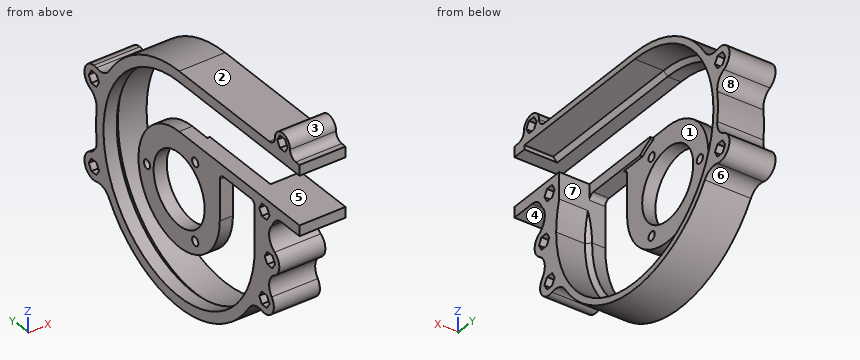
```python
from build123d import *

# Parameters (mm, degrees)
SKETCH_2_W           = 17.5
SKETCH_2_H           = 4
EXTRUDE_1_DEPTH      = 6
SKETCH_6_R           = 13.5
SKETCH_6_R_2         = 1.65
EXTRUDE_2_DEPTH      = 5
FILLET_1_R           = 2
EXTRUDE_START        = -17.5
SKETCH_7_R           = 5
EXTRUDE_3_DEPTH      = 17.5
FILLET_2_R           = 6
CUT_EXTRUDE_1_DEPTH  = 72.072146443
SKETCH_9_W           = 17.5
SKETCH_9_H           = 4
EXTRUDE_4_DEPTH      = 11.4
FILLET_3_R           = 5
EXTRUDE_5_DEPTH      = 0.28
EXTRUDE_5_DEPTH_BACK = 5
SKETCH_10_W          = 17.5
SKETCH_10_H          = 4
SKETCH_11_R          = 4
EXTRUDE_6_DEPTH      = 17.5
FILLET_4_R           = 3


with BuildPart() as part:
    # Sweep 1: sweep along a path in 草图1
    with BuildLine(Plane(origin=(0, 0, 0), x_dir=(0, 0, -1), z_dir=(1, 0, 0))) as sweep_1_path:
        Line((-44, -52), (-44, 0))
        ThreePointArc((-44, 0), (31.112698372, 31.112698372), (0, -44))
        Line((0, -44), (-17.5, -44))
        Line((-17.5, -44), (-17.5, -52))
    # 草图2 → Sweep 1 (sweep)
    with BuildSketch(Plane(origin=(0, -52, 0), x_dir=(1, 0, 0), z_dir=(0, 1, 0))):
        with Locations((8.75, -42)):
            Rectangle(SKETCH_2_W, SKETCH_2_H)
    sweep(path=sweep_1_path.line, transition=Transition.RIGHT)

    # Sweep 1 2: sweep along a path in 草图4
    with BuildLine(Plane.ZY) as sweep_1_2_path:
        Line((44, -52), (44, 0))
        ThreePointArc((44, 0), (-31.112698372, 31.112698372), (0, -44))
        ThreePointArc((0, -44), (12.692125838, -42.129680057), (24.3052364, -36.677724623))
    # 草图3 → Sweep 1 2 (sweep, cut)
    with BuildSketch(Plane(origin=(0, -52, 0), x_dir=(1, 0, 0), z_dir=(0, 1, 0))):
        Polygon((17.5, -40), (5, -40), (6.6, -41.6), (17.5, -41.6), align=None)
    sweep(path=sweep_1_2_path.line, mode=Mode.SUBTRACT)

    # 草图5 → 凸台-拉伸1 (add)
    with BuildSketch(Plane.ZY):
        with BuildLine():
            Line((21.5, -40), (21.5, -8.077747211))
            ThreePointArc((21.5, -8.077747211), (21.091287093, -7.586151171), (20.533333333, -7.898241717))
            ThreePointArc((20.533333333, -7.898241717), (19.209784895, -10.723066925), (17.5, -13.332291626))
            Line((17.5, -13.332291626), (17.5, -40))
            Line((17.5, -40), (21.5, -40))
        make_face()
    extrude(amount=-EXTRUDE_1_DEPTH)

    # 草图6 → 凸台-拉伸2 (add)
    with BuildSketch(Plane.ZY):
        with BuildLine():
            Line((21.5, -21.5), (21.5, -8.077747211))
            Line((21.5, -8.077747211), (21.5, 0))
            ThreePointArc((21.5, 0), (-15.202795796, 15.202795796), (0, -21.5))
            Line((0, -21.5), (21.5, -21.5))
        make_face()
        Circle(SKETCH_6_R, mode=Mode.SUBTRACT)
        with Locations((0, 17)):
            Circle(SKETCH_6_R_2, mode=Mode.SUBTRACT)
        with Locations((14.722431864, -8.5)):
            Circle(SKETCH_6_R_2, mode=Mode.SUBTRACT)
        with Locations((-14.722431864, -8.5)):
            Circle(SKETCH_6_R_2, mode=Mode.SUBTRACT)
    extrude(amount=-EXTRUDE_2_DEPTH)

    # 圆角1
    fillet_1_edges = [part.edges().sort_by_distance(p)[0] for p in [
        (3, -40, 17.5),
        (2.5, -21.5, 17.5),
    ]]
    fillet(fillet_1_edges, radius=FILLET_1_R)

    # 草图7 → 凸台-拉伸3 (add)
    # profile 1 of 7: a face of its own
    with BuildSketch(Plane.ZY.offset(EXTRUDE_START)):
        with BuildLine():
            ThreePointArc((-11.41696688, -45.105245798), (-11.647855738, -43.60338731), (-12.319198447, -42.240233778))
            ThreePointArc((-12.319198447, -42.240233778), (-15.048886306, -41.346475315), (-17.714445389, -40.276524485))
            ThreePointArc((-17.714445389, -40.276524485), (-20.865936265, -47.387058983), (-13.252416867, -48.976372665))
            ThreePointArc((-13.252416867, -48.976372665), (-11.899071902, -47.247353398), (-11.41696688, -45.105245798))
        make_face()
        Polygon((-14.06696688, -46.46201893), (-16.41696688, -47.818792063), (-18.76696688, -46.46201893), (-18.76696688, -43.748472665), (-16.41696688, -42.391699533), (-14.06696688, -43.748472665), align=None, mode=Mode.SUBTRACT)
    # profile 2 of 7: a face of its own
    with BuildSketch(Plane.ZY.offset(EXTRUDE_START)):
        with BuildLine():
            ThreePointArc((-4.29770766, -50.555329502), (-4.888687372, -46.950840441), (-2.870750936, -43.90625))
            ThreePointArc((-2.870750936, -43.90625), (-7.640519817, -43.331541133), (-12.319198447, -42.240233778))
            ThreePointArc((-12.319198447, -42.240233778), (-11.647855738, -43.60338731), (-11.41696688, -45.105245798))
            ThreePointArc((-11.41696688, -45.105245798), (-11.899071902, -47.247353398), (-13.252416867, -48.976372665))
            ThreePointArc((-13.252416867, -48.976372665), (-8.413067787, -47.712878387), (-4.29770766, -50.555329502))
        make_face()
    # profile 3 of 7: a face of its own
    with BuildSketch(Plane.ZY.offset(EXTRUDE_START)):
        with BuildLine():
            ThreePointArc((5, -48), (4.472135955, -45.763932023), (3, -44))
            ThreePointArc((3, -44), (1.58113883, -43.25658351), (0, -43))
            Line((0, -43), (0, -44))
            ThreePointArc((0, -44), (-1.436140662, -43.976556254), (-2.870750936, -43.90625))
            ThreePointArc((-2.870750936, -43.90625), (-4.888687372, -46.950840441), (-4.29770766, -50.555329502))
            ThreePointArc((-4.29770766, -50.555329502), (0, -53), (4.29770766, -50.555329502))
            ThreePointArc((4.29770766, -50.555329502), (4.821231083, -49.325039942), (5, -48))
        make_face()
        Polygon((-2.35, -46.643226867), (0, -45.286453735), (2.35, -46.643226867), (2.35, -49.356773133), (0, -50.713546265), (-2.35, -49.356773133), align=None, mode=Mode.SUBTRACT)
    # profile 4 of 7: a face of its own
    with BuildSketch(Plane.ZY.offset(EXTRUDE_START)):
        with BuildLine():
            Line((11.540653546, -44), (3, -44))
            ThreePointArc((3, -44), (4.472135955, -45.763932023), (5, -48))
            ThreePointArc((5, -48), (4.821231083, -49.325039942), (4.29770766, -50.555329502))
            ThreePointArc((4.29770766, -50.555329502), (8.413067787, -47.712878387), (13.252416867, -48.976372665))
            ThreePointArc((13.252416867, -48.976372665), (11.688865563, -46.731609207), (11.540653546, -44))
        make_face()
    # profile 5 of 7: a face of its own
    with BuildSketch(Plane.ZY.offset(EXTRUDE_START)):
        with Locations((16.41696688, -45.105245798)):
            Circle(SKETCH_7_R)
        Polygon((18.76696688, -46.46201893), (16.41696688, -47.818792063), (14.06696688, -46.46201893), (14.06696688, -43.748472665), (16.41696688, -42.391699533), (18.76696688, -43.748472665), align=None, mode=Mode.SUBTRACT)
    # profile 6 of 7: a face of its own
    with BuildSketch(Plane.ZY.offset(EXTRUDE_START)):
        with BuildLine():
            ThreePointArc((-11.41696688, 45.105245798), (-19.459384295, 49.07307849), (-17.714445389, 40.276524485))
            ThreePointArc((-17.714445389, 40.276524485), (-15.048886306, 41.346475315), (-12.319198447, 42.240233778))
            ThreePointArc((-12.319198447, 42.240233778), (-11.647855738, 43.60338731), (-11.41696688, 45.105245798))
        make_face()
        Polygon((-18.76696688, 43.748472665), (-18.76696688, 46.46201893), (-16.41696688, 47.818792063), (-14.06696688, 46.46201893), (-14.06696688, 43.748472665), (-16.41696688, 42.391699533), align=None, mode=Mode.SUBTRACT)
    # profile 7 of 7: a face of its own
    with BuildSketch(Plane.ZY.offset(EXTRUDE_START)):
        with BuildLine():
            ThreePointArc((21.41696688, 45.105245798), (14.915108391, 49.874356939), (12.319198447, 42.240233778))
            ThreePointArc((12.319198447, 42.240233778), (15.048886306, 41.346475315), (17.714445389, 40.276524485))
            ThreePointArc((17.714445389, 40.276524485), (20.384799572, 42.062828383), (21.41696688, 45.105245798))
        make_face()
        Polygon((14.06696688, 46.46201893), (16.41696688, 47.818792063), (18.76696688, 46.46201893), (18.76696688, 43.748472665), (16.41696688, 42.391699533), (14.06696688, 43.748472665), align=None, mode=Mode.SUBTRACT)
    extrude(amount=EXTRUDE_3_DEPTH)

    # 圆角2
    # the kernel refuses this fillet: 6 mm, written as the material it adds along each edge
    with BuildSketch(Plane(origin=(17.5, 40.276524485, -17.714445389), x_dir=(0, -0.4726837072692949, -0.8812321560645388), z_dir=(-1, 0, 0)), Plane(origin=(17.5, 42.240233778, 12.319198447), x_dir=(0, 0.20434838386912327, -0.978898226584397), z_dir=(-1, 0, 0))) as fillet_2_piece_1:
        with BuildLine():
            CenterArc((7.322424831, -5.98176794), FILLET_2_R, 94.467760731, 73.250864603)
            Line((1.459736191, -4.705491359), (1.342482418, -4.679965828))
            ThreePointArc((1.342482418, -4.679965828), (1.235040355, -2.196031285), (-0.082220104, -0.087406261))
            Line((-0.082220104, -0.087406261), (0.009347776, 0.119635359))
            ThreePointArc((0.009347776, 0.119635359), (3.427518006, -0.013701771), (6.845688236, 0.119635359))
            Line((6.845688236, 0.119635359), (6.855036012, 0))
        make_face()
    extrude(amount=17.5)
    with BuildSketch(Plane(origin=(17.5, 42.240233778, -12.319198447), x_dir=(0, 0.20434838386906956, 0.9788982265844082), z_dir=(-1, 0, 0)), Plane(origin=(17.5, 40.276524485, 17.714445389), x_dir=(0, -0.47268370726929204, 0.8812321560645403), z_dir=(-1, 0, 0)), Plane(origin=(17.5, -40.276524485, -17.714445389), x_dir=(0, 0.47268370726929143, -0.8812321560645405), z_dir=(-1, 0, 0))) as fillet_2_piece_2:
        with BuildLine():
            CenterArc((7.322424831, 5.98176794), FILLET_2_R, 192.281374666, 73.250864603)
            Line((1.459736191, 4.705491359), (1.342482418, 4.679965828))
            ThreePointArc((1.342482418, 4.679965828), (1.235040355, 2.196031285), (-0.082220104, 0.087406261))
            Line((-0.082220104, 0.087406261), (0.009347776, -0.119635359))
            ThreePointArc((0.009347776, -0.119635359), (3.427518006, 0.013701771), (6.845688236, -0.119635359))
            Line((6.845688236, -0.119635359), (6.855036012, 0))
        make_face()
    extrude(amount=17.5)
    with BuildSketch(Plane(origin=(0, -49.986540632, 17.5), x_dir=(0, -1, 0), z_dir=(1, 0, 0))) as fillet_2_piece_3:
        with BuildLine():
            CenterArc((5.420881339, 4.938570189), FILLET_2_R, 200.518106547, 34.877722735)
            Line((-0.198487483, 2.83554997), (-0.310874859, 2.793489565))
            ThreePointArc((-0.310874859, 2.793489565), (-0.013206953, 1.423797529), (-0.117151076, 0.025992795))
            Line((-0.117151076, 0.025992795), (0, -0.12))
            ThreePointArc((0, -0.12), (1.006729684, -0.12), (1.945310928, -0.098771404))
            Line((1.945310928, -0.098771404), (2.013459368, 0))
        make_face()
    extrude(amount=17.5)

    # 草图8 → 切除-拉伸1 (cut, through all)
    with BuildSketch(Plane(origin=(17.5, 0, 0), x_dir=(0, 0, -1), z_dir=(1, 0, 0))):
        Polygon((-14.06696688, -46.46201893), (-14.06696688, -43.748472665), (-16.41696688, -42.391699533), (-18.76696688, -43.748472665), (-18.76696688, -46.46201893), (-16.41696688, -47.818792063), align=None)
    extrude(amount=-CUT_EXTRUDE_1_DEPTH, mode=Mode.SUBTRACT)

    # 草图9 → 凸台-拉伸4 (add)
    with BuildSketch(Plane.XZ.offset(52)):
        with Locations((8.75, 19.5)):
            Rectangle(SKETCH_9_W, SKETCH_9_H)
        Polygon((6.6, 41.6), (17.5, 41.6), (17.5, 44), (0, 44), (0, 40), (5, 40), align=None)
    extrude(amount=EXTRUDE_4_DEPTH)

    # 圆角3
    fillet_3_edges = [part.edges().sort_by_distance(p)[0] for p in [
        (8.75, -52, 17.5),
    ]]
    fillet(fillet_3_edges, radius=FILLET_3_R)

    # 草图10 → 凸台-拉伸5 (add, two sides: drawn at the far end of the back side and taken through both)
    with BuildSketch(Plane.XZ.offset(63.4).offset(-EXTRUDE_5_DEPTH_BACK)):
        with Locations((8.75, 42)):
            Rectangle(SKETCH_10_W, SKETCH_10_H)
        with Locations((8.75, 19.5)):
            Rectangle(SKETCH_10_W, SKETCH_10_H)
    extrude(amount=EXTRUDE_5_DEPTH + EXTRUDE_5_DEPTH_BACK)

    # 草图11 → 凸台-拉伸6 (add)
    with BuildSketch(Plane(origin=(17.5, 0, 0), x_dir=(0, 0, -1), z_dir=(1, 0, 0))):
        with Locations((-47, -54.68)):
            Circle(SKETCH_11_R)
        Polygon((-44.65, -53.323226867), (-47, -51.966453735), (-49.35, -53.323226867), (-49.35, -56.036773133), (-47, -57.393546265), (-44.65, -56.036773133), align=None, mode=Mode.SUBTRACT)
    extrude(amount=-EXTRUDE_6_DEPTH)

    # 圆角4
    fillet_4_edges = [part.edges().sort_by_distance(p)[0] for p in [
        (8.75, -52.034248689, 44),
        (8.75, -57.325751311, 44),
    ]]
    fillet(fillet_4_edges, radius=FILLET_4_R)


solid = part.part
```
For this review, take the finished solid that the model builds, in its own axes (mm). Face numbers are marked on the shaded views. A direction names the side the tool comes from. Give positions to 0.01 mm unless a question says otherwise; leave off trailing zeros. One line per item, written item: value. Start each with the question number.
Q1. Draft analysis for pull direction Y (two halves, no side actions). For the marked faces 1, 2 and 3, state which applies: released by +Y, released by -Y, zero draft, split by the parting line, or undercut.
Q2. Machinability: for the marked faces 4, 5, 6, 7 and 8, which of the approach directions +Z, -Z, +X, -X, +Y, -Y give a long, thin tool a straight path to every point of the face, cutting with its end or side? Answer none if there is none.
Q3. Clearance check with flat-ended pins moving along their axes: pin 1 Ø2 at (y, z) = (-8.5, 14.72) entering from -X; pin 2 Ø4 at (x, z) = (9.5, -10.5) entering from -Y; pin 3 Ø1.5 at (x, y) = (7, -10.5) entering from +Z; pin 4 Ø2 at (x, z) = (3, -5) entering from +Y. State where each tip first meets the part, or that it passes through.
Q4. For L1, parallel to Z at x = 1.5, y = 16; L2, parallel to Z at x = 12.5, y = 0; L3, parallel to Z at x = 3.75, y = -23, list the stretches that pass through material, from the lowest coordinate up.
Q5. Add section A-A (z = -7). Count the separate pieces of the cut face and the enclosed holes in it, and give its area (3 significant figures).
Reply:
1. face 1: undercut
1. face 2: zero draft
1. face 3: split by the parting line
2. face 4: -Z, +X, -X, -Y
2. face 5: +X, -X, -Y
2. face 6: -Z, +X, -X
2. face 7: +X
2. face 8: +X, -X, +Y
3. pin 1: through
3. pin 2: y = -48.45
3. pin 3: z = 44
3. pin 4: y = 43.82
4. L1: -40.99 to -36.66, -14.36 to -1.31, 1.31 to 14.36, 36.66 to 40.99
4. L2: -44 to -41.6, 41.6 to 44
4. L3: -37.51 to -32.73, 17.44 to 21.5, 40 to 44
5. separate pieces: 4
5. enclosed holes: 0
5. area: 277 mm²
